Check sheet for the modelled part. Datum: model origin and axes. Units: mm. Face numbers are marked on the shaded views. A direction names the side the tool comes from. Coordinates: 2 decimals unless noted, no trailing zeros. Loops run counter-clockwise (first coordinate to the right, second up) from the corner with the lowest first, then second, coordinate; pieces in that order, holes last. Notation, with made-up numbers: M -27,13 L 25,13 A14 cw 25,24 Z; hole C 45.25,-8.5 d6. An arc over 180 degrees is marked long. Return JSON: item names as keys, results as strings.
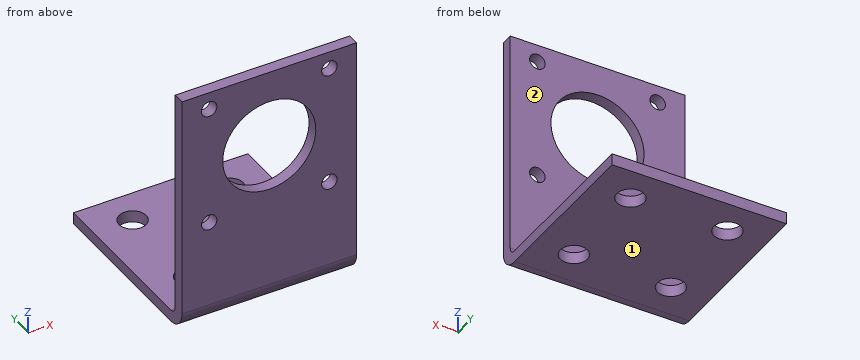
from build123d import *

# Parameters (mm, degrees)
BOSS_EXTRUDE1_DEPTH = 45
FILLET1_R           = 2
FILLET2_R           = 5
CUT_EXTRUDE1_REACH  = 93.093
SKETCH2_R           = 2
SKETCH2_R_2         = 12
SKETCH3_R           = 3.5
CUT_EXTRUDE2_DEPTH  = 90.044932478


with BuildPart() as part:
    # Sketch1 → Boss-Extrude1 (new body)
    with BuildSketch(Plane(origin=(0, 0, 0), x_dir=(0, 0, -1), z_dir=(1, 0, 0))):
        Polygon((0, 0), (0, 48), (-3, 48), (-3, 3), (-63, 3), (-63, 0), align=None)
    extrude(amount=BOSS_EXTRUDE1_DEPTH)

    # Fillet1
    fillet1_edges = [part.edges().sort_by_distance(p)[0] for p in [
        (22.5, 3, 3),
    ]]
    fillet(fillet1_edges, radius=FILLET1_R)

    # Fillet2
    fillet2_edges = [part.edges().sort_by_distance(p)[0] for p in [
        (22.5, 0, 0),
    ]]
    fillet(fillet2_edges, radius=FILLET2_R)

    # Sketch2 → Cut-Extrude1 (cut, up to next)
    with BuildSketch(Plane.XZ, mode=Mode.PRIVATE) as cut_extrude1_sk1:
        with Locations(Location((38, 58.5, 0), (0, 0, 270))):
            Circle(SKETCH2_R)
    cut_extrude1_tool1 = extrude(cut_extrude1_sk1.sketch, amount=-CUT_EXTRUDE1_REACH, mode=Mode.PRIVATE) & part.part
    # Sketch2 → Cut-Extrude1 (cut, up to next)
    with BuildSketch(Plane.XZ, mode=Mode.PRIVATE) as cut_extrude1_sk2:
        with Locations(Location((38, 27.5, 0), (0, 0, 270))):
            Circle(SKETCH2_R)
    cut_extrude1_tool2 = extrude(cut_extrude1_sk2.sketch, amount=-CUT_EXTRUDE1_REACH, mode=Mode.PRIVATE) & part.part
    # Sketch2 → Cut-Extrude1 (cut, up to next)
    with BuildSketch(Plane.XZ, mode=Mode.PRIVATE) as cut_extrude1_sk3:
        with Locations(Location((7, 58.5, 0), (0, 0, 270))):
            Circle(SKETCH2_R)
    cut_extrude1_tool3 = extrude(cut_extrude1_sk3.sketch, amount=-CUT_EXTRUDE1_REACH, mode=Mode.PRIVATE) & part.part
    # Sketch2 → Cut-Extrude1 (cut, up to next)
    with BuildSketch(Plane.XZ, mode=Mode.PRIVATE) as cut_extrude1_sk4:
        with Locations(Location((7, 27.5, 0), (0, 0, 270))):
            Circle(SKETCH2_R)
    cut_extrude1_tool4 = extrude(cut_extrude1_sk4.sketch, amount=-CUT_EXTRUDE1_REACH, mode=Mode.PRIVATE) & part.part
    # Sketch2 → Cut-Extrude1 (cut, up to next)
    with BuildSketch(Plane.XZ, mode=Mode.PRIVATE) as cut_extrude1_sk5:
        with Locations(Location((22.5, 43, 0), (0, 0, 270))):
            Circle(SKETCH2_R_2)
    cut_extrude1_tool5 = extrude(cut_extrude1_sk5.sketch, amount=-CUT_EXTRUDE1_REACH, mode=Mode.PRIVATE) & part.part
    add(cut_extrude1_tool1.solids().sort_by_distance((38, 0, 58.5))[0], mode=Mode.SUBTRACT)
    add(cut_extrude1_tool2.solids().sort_by_distance((38, 0, 27.5))[0], mode=Mode.SUBTRACT)
    add(cut_extrude1_tool3.solids().sort_by_distance((7, 0, 58.5))[0], mode=Mode.SUBTRACT)
    add(cut_extrude1_tool4.solids().sort_by_distance((7, 0, 27.5))[0], mode=Mode.SUBTRACT)
    add(cut_extrude1_tool5.solids().sort_by_distance((22.5, 0, 43))[0], mode=Mode.SUBTRACT)

    # Sketch3 → Cut-Extrude2 (cut, through all)
    with BuildSketch(Plane.XY.offset(3)):
        with Locations((35, 39)):
            Circle(SKETCH3_R)
        with Locations((35, 14)):
            Circle(SKETCH3_R)
        with Locations((10, 39)):
            Circle(SKETCH3_R)
        with Locations((10, 14)):
            Circle(SKETCH3_R)
    extrude(amount=-CUT_EXTRUDE2_DEPTH, mode=Mode.SUBTRACT)


solid = part.part
1) Set-up check for the marked faces 1 and 2: record each of +Z, -Z, +X, -X, +Y, -Y from which the full face is reachable in a straight line by a thin tool's end or side.
Answers:
{"face 1": "-Z, +X, -X, +Y, -Y", "face 2": "+Z, +X, -X, +Y"}
2) Section check A-A on y = 39. Record the cut outline in (x, z), then the cut area to 3 significant figures.
Answers:
{"outline": "M 0,0 L 6.5,0 L 6.5,3 L 0,3 Z; M 13.5,0 L 31.5,0 L 31.5,3 L 13.5,3 Z; M 38.5,0 L 45,0 L 45,3 L 38.5,3 Z", "area": "93.0 mm²"}
3) Go/stop test with flat-tipped pins: pin 1 Ø9 at (x, y) = (10, 14) entering from +Z; pin 2 Ø3.5 at (x, z) = (38, 58.5) entering from -Y; pin 3 Ø13.5 at (x, z) = (14.5, 25) entering from +Y. Record where each tip stops, or that it passes through.
Answers:
{"pin 1": "z = 3", "pin 2": "through", "pin 3": "y = 3"}
4) Section check C-C on x = 22.5. Record the cut outline in (y, z).
Answers:
{"outline": "M 0,5 A5 ccw 5,0 L 48,0 L 48,3 L 5,3 A2 cw 3,5 L 3,31 L 0,31 Z; M 0,55 L 3,55 L 3,63 L 0,63 Z"}
5) Section check D-D on z = 33.5. Record the cut outline in (x, y), then the cut area to 3 significant figures.
Answers:
{"outline": "M 0,0 L 15.17,0 L 15.17,3 L 0,3 Z; M 29.83,0 L 45,0 L 45,3 L 29.83,3 Z", "area": "91.0 mm²"}
6) Section check B-B on z = 58.5. Record the cut outline in (x, y).
Answers:
{"outline": "M 0,0 L 5,0 L 5,3 L 0,3 Z; M 9,0 L 36,0 L 36,3 L 9,3 Z; M 40,0 L 45,0 L 45,3 L 40,3 Z"}
7) Scan lines: line 1 along X through (y, z) = (0.75, 58.5); line 2 along X through (y, z) = (1.9, 43); line 3 along Y through (x, z) = (10, 1.5). Record each from-to range of solid material in increasing order. Write a range as [from, to].
Answers:
{"line 1": "[0, 5], [9, 36], [40, 45]", "line 2": "[0, 10.5], [34.5, 45]", "line 3": "[1.43, 10.5], [17.5, 35.5], [42.5, 48]"}
